Read the model definition and answer for the solid it produces. Units are mm, in the model's axes. Face numbers are marked on the shaded views. Coordinates: 2 decimals unless noted, no trailing zeros. Loops run counter-clockwise (first coordinate to the right, second up) from the corner with the lowest first, then second, coordinate; pieces in that order, holes last. Notation, with made-up numbers: M 26,37 L 73,37 A13 ccw 73,41 Z; hole C 16.25,-4 d11. An arc over 180 degrees is marked long. Use one line per item in the form item = value. Start each with the question number.
1. Find the intervals of material crossed by probe 1 along Y at (x, z) = (568, 512.5), in increasing order. Write a range as [from, to].
2. For a pull along X with two mould halves and no side action, classify the marked faces 1, 2 and 3 as released by +X, released by -X, zero draft, split by the parting line, or undercut.
3. Flat-ended cylindrical pins translate along their axes: pin 1 (7.5 mm diameter, centred on y = -8.5, z = 1336.5, fed in from +X); pin 2 (7.5 mm diameter, centred on y = -11, z = 383.5, fed in from +X); pin 3 (7.5 mm diameter, centred on x = 250, y = -15.5, fed in from -Z). Find the tip coordinate at first contact, or state that the pin passes through.
4. The part is cut by section A-A (x = 422.5). Give the vertices of the cut face in (y, z) (3 decimals), plus the area to 3 significant figures.
from build123d import *

# Parameters (mm, degrees)
F0_W     = 831.85
F0_H     = 889
F1_DEPTH = 1768.475
F2_W     = 301.625
F2_H     = 1143
F2_W_2   = 679.45
F2_H_2   = 346.075
F3_DEPTH = 25.4


with BuildPart() as f1:
    # F0 (on Top) → F1 (new body)
    with BuildSketch(Plane.XY):
        with Locations((415.925, 444.5)):
            Rectangle(F0_W, F0_H)
    extrude(amount=F1_DEPTH)

    # F2 (on face) → F3 (join)
    with BuildSketch(Plane.XZ):
        with Locations((227.0125, 1120.775)):
            Rectangle(F2_W, F2_H)
        with Locations((604.8375, 1120.775)):
            Rectangle(F2_W, F2_H)
        with Locations((415.925, 300.0375)):
            Rectangle(F2_W_2, F2_H_2)
    extrude(amount=F3_DEPTH)


solid = f1.part
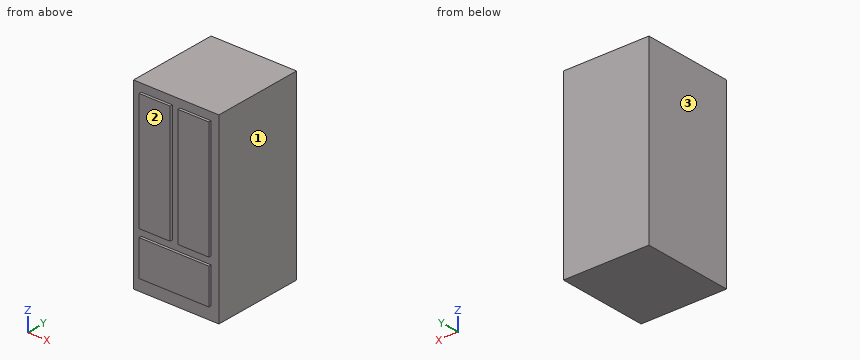
Computed values:
q1.probe_1 = [0, 889]
q2.face_1 = released by +X
q2.face_2 = zero draft
q2.face_3 = released by -X
q3.pin_1 = 755.65
q3.pin_2 = 755.65
q3.pin_3 = 127
q4.outline = M -25.4,127 L 0,127 L 0,0 L 889,0 L 889,1768.475 L 0,1768.475 L 0,473.075 L -25.4,473.075 Z
q4.area = 1,580,000 mm²
